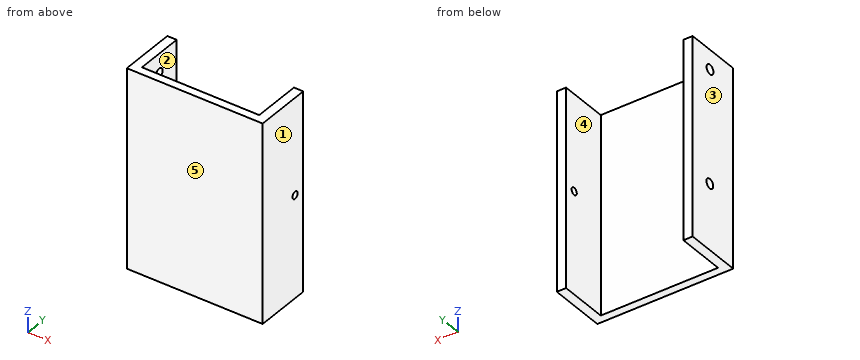
from build123d import *

# Parameters (mm, degrees)
BOSS_EXTRUDE3_DEPTH = 111.125
SKETCH4_R           = 2.667
CUT_EXTRUDE1_DEPTH  = 136.634929771
SKETCH5_R           = 2.667
CUT_EXTRUDE2_DEPTH  = 136.634929771
SKETCH6_R           = 2.032
CUT_EXTRUDE3_DEPTH  = 136.634929771


with BuildPart() as part:
    # Sketch2 → Boss-Extrude3 (new body)
    with BuildSketch(Plane.XY):
        Polygon((-38.1, 0), (38.1, 0), (38.1, 31.75), (32.893, 31.75), (32.893, 4.5974), (-32.893, 4.5974), (-32.893, 31.75), (-38.1, 31.75), align=None)
    extrude(amount=BOSS_EXTRUDE3_DEPTH)

    # Sketch4 → Cut-Extrude1 (cut, through all)
    with BuildSketch(Plane(origin=(-32.893, 0, 0), x_dir=(0, 0, -1), z_dir=(1, 0, 0))):
        with Locations((-36.83, 18.288)):
            Circle(SKETCH4_R)
    extrude(amount=-CUT_EXTRUDE1_DEPTH, mode=Mode.SUBTRACT)

    # Sketch5 → Cut-Extrude2 (cut, through all)
    with BuildSketch(Plane(origin=(-32.893, 0, 0), x_dir=(0, 0, -1), z_dir=(1, 0, 0))):
        with Locations((-100.203, 18.163390835)):
            Circle(SKETCH5_R)
    extrude(amount=-CUT_EXTRUDE2_DEPTH, mode=Mode.SUBTRACT)

    # Sketch6 → Cut-Extrude3 (cut, through all)
    with BuildSketch(Plane.ZY.offset(-32.893)):
        with Locations((57.15, 25.4)):
            Circle(SKETCH6_R)
    extrude(amount=-CUT_EXTRUDE3_DEPTH, mode=Mode.SUBTRACT)


solid = part.part
Geometry: final body of the model. Coordinates: model frame, mm. Face numbers are marked on the shaded views. A direction names the side the tool comes from. Round coordinates to 2 decimals unless told otherwise and drop trailing zeros. Order: outer loops, then holes, each group sorted by start corner. A loop starts at its lowest first (then second) coordinate and runs counter-clockwise, first axis right, second up. Notation, with made-up numbers: (46, 60) -> (52, 60) arc R17 ccw to (52, 68) -> close; hole circle Ø11 at (7, -37.5). An arc over 180 degrees is marked (long way). Put each result on its own line as item: value. Start each with the question number.
Q1. Section C-C on y = 10.5. Return the cut outline in (x, z) (3 decimals), and give its area (3 significant figures).
Q2. Line query: probe 1 along X at (y, z) = (26.5, 64.5); probe 2 along X at (y, z) = (26.5, 57.5); probe 3 along Y at (x, z) = (18, 17). Output: solid intervals per line, ascending.
Q3. Reachability of the marked faces 4 and 5 from +Z, -Z, +X, -X, +Y, -Y: full face, straight path, thin tool, end or side. Return the list, or none.
Q4. Pull-direction query (X, two-part tool) for the marked faces 1, 2 and 3; classes: +X half, -X half, draft (parallel to the pull), parting line (faces both ways), or undercut.
Q5. Section D-D on y = 19.5. Return the cut outline in (x, z) (3 decimals), and give its area (3 significant figures).
Q6. Section B-B on y = 25.4. Return the cut outline in (x, z) (3 decimals).
Q7. First-contact query: pin 1 (12 mm diameter, centred on x = -25, y = 22, fed in from +Z). Flat tip, straight axial feed; report the tip coordinate or a pass-through.
Q8. Section A-A on z = 57.15. Return the cut outline in (x, y).
Ans:
1. outline: (-38.1, 0) -> (-32.893, 0) -> (-32.893, 111.125) -> (-38.1, 111.125) -> close; (32.893, 0) -> (38.1, 0) -> (38.1, 111.125) -> (32.893, 111.125) -> close
1. area: 1,160 mm2
2. probe 1: x = -38.1 to -32.89, 32.89 to 38.1
2. probe 2: x = -38.1 to -32.89
2. probe 3: y = 0 to 4.6
3. face 4: +Z, -Z, +Y
3. face 5: +Z, -Z, +X, -X, -Y
4. face 1: +X half
4. face 2: undercut
4. face 3: -X half
5. outline: (-38.1, 0) -> (-32.893, 0) -> (-32.893, 34.454) -> (-38.1, 34.454) -> close; (-38.1, 39.206) -> (-32.893, 39.206) -> (-32.893, 97.895) -> (-38.1, 97.895) -> close; (-38.1, 102.511) -> (-32.893, 102.511) -> (-32.893, 111.125) -> (-38.1, 111.125) -> close; (32.893, 0) -> (38.1, 0) -> (38.1, 111.125) -> (32.893, 111.125) -> close
5. area: 1,110 mm2
6. outline: (-38.1, 0) -> (-32.893, 0) -> (-32.893, 111.125) -> (-38.1, 111.125) -> close; (32.893, 0) -> (38.1, 0) -> (38.1, 55.118) -> (32.893, 55.118) -> close; (32.893, 59.182) -> (38.1, 59.182) -> (38.1, 111.125) -> (32.893, 111.125) -> close
7. pin 1: passes through
8. outline: (-38.1, 0) -> (38.1, 0) -> (38.1, 23.37) -> (32.89, 23.37) -> (32.89, 4.6) -> (-32.89, 4.6) -> (-32.89, 31.75) -> (-38.1, 31.75) -> close; (32.89, 27.43) -> (38.1, 27.43) -> (38.1, 31.75) -> (32.89, 31.75) -> close
